from build123d import *

# Parameters (mm, degrees)
SKETCH1_R           = 1.5
SKETCH1_R_2         = 1
BOSS_EXTRUDE1_DEPTH = 4
FILLET1_R           = 10
FILLET2_R           = 10
FILLET3_R           = 10
FILLET4_R           = 10


with BuildPart() as part:
    # Sketch1 → Boss-Extrude1 (new body)
    with BuildSketch(Plane(origin=(0, 0, 0), x_dir=(1, 0, 0), z_dir=(0, 1, 0))):
        Polygon((-43.595803766, -205.807188304), (-22.135109681, -203.371959758), (-24.298008335, -184.311199966), (34.130185477, -177.681125241), (36.293084131, -196.741885032), (57.753778216, -194.306656487), (62.409879754, -235.339014996), (-38.939702228, -246.839546813), align=None)
        with Locations(Location((-29.093140713, -209.445179895, 0), (0, 0, 270))):
            Circle(SKETCH1_R, mode=Mode.SUBTRACT)
        with Locations(Location((44.434987391, -201.101656812, 0), (0, 0, 90))):
            Circle(SKETCH1_R, mode=Mode.SUBTRACT)
        with Locations(Location((11.278933321, -237.069365642, 0), (0, 0, 270))):
            Circle(SKETCH1_R, mode=Mode.SUBTRACT)
        with Locations(Location((-9.197768444, -205.174739373, 0), (0, 0, 270))):
            Circle(SKETCH1_R_2, mode=Mode.SUBTRACT)
        with Locations(Location((-11.22676603, -187.293996073, 0), (0, 0, 270))):
            Circle(SKETCH1_R_2, mode=Mode.SUBTRACT)
        with Locations(Location((22.059616288, -183.516860623, 0), (0, 0, 270))):
            Circle(SKETCH1_R_2, mode=Mode.SUBTRACT)
        with Locations(Location((24.088613874, -201.397603923, 0), (0, 0, 270))):
            Circle(SKETCH1_R_2, mode=Mode.SUBTRACT)
    extrude(amount=BOSS_EXTRUDE1_DEPTH)

    # Fillet1
    fillet1_edges = [part.edges().sort_by_distance(p)[0] for p in [
        (-38.939702228, 2, 246.839546813),
    ]]
    fillet(fillet1_edges, radius=FILLET1_R)

    # Fillet2
    fillet2_edges = [part.edges().sort_by_distance(p)[0] for p in [
        (62.409879754, 2, 235.339014996),
    ]]
    fillet(fillet2_edges, radius=FILLET2_R)

    # Fillet3
    fillet3_edges = [part.edges().sort_by_distance(p)[0] for p in [
        (57.753778216, 2, 194.306656487),
    ]]
    fillet(fillet3_edges, radius=FILLET3_R)

    # Fillet4
    fillet4_edges = [part.edges().sort_by_distance(p)[0] for p in [
        (-43.595803766, 2, 205.807188304),
    ]]
    fillet(fillet4_edges, radius=FILLET4_R)


solid = part.part
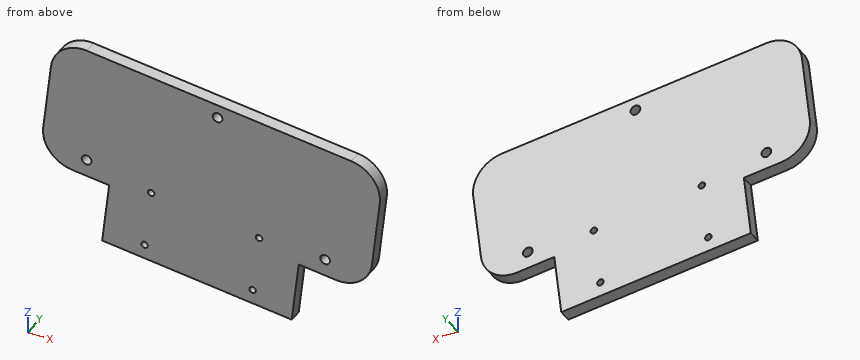
Part model, mm, in its own coordinate system. Coordinates: 2 decimals unless noted, no trailing zeros. Order: outer loops, then holes, each group sorted by start corner. A loop starts at its lowest first (then second) coordinate and runs counter-clockwise, first axis right, second up.
(1) Slice it at A-A, the plane y = 2.95. Write the cut outline in (x, z), and give its area (3 significant figures).
Check sheet entries:
outline: (-42.47, 215.74) arc R10 ccw to (-33.66, 204.68) - (-22.14, 203.37) - (-24.3, 184.31) - (34.13, 177.68) - (36.29, 196.74) - (47.82, 195.43) arc R10 ccw to (58.88, 204.24) - (61.28, 225.4) arc R10 ccw to (52.47, 236.47) - (-29, 245.71) arc R10 ccw to (-40.07, 236.9) - close; hole circle Ø3 at (-29.09, 209.45); hole circle Ø2 at (-11.23, 187.29); hole circle Ø2 at (-9.2, 205.17); hole circle Ø3 at (11.28, 237.07); hole circle Ø2 at (22.06, 183.52); hole circle Ø2 at (24.09, 201.4); hole circle Ø3 at (44.43, 201.1)
area: 5,220 mm2
(2) Pin check, flat tips, straight feed: pin 1 Ø1.5 at (y, z) = (2, 216) entering from -X; pin 2 Ø2 at (x, y) = (7, 1.5) entering from -Z; pin 3 Ø2 at (y, z) = (1, 221) entering from -X. Stop position of each tip, or through.
Check sheet entries:
pin 1: stops at x = -42.51
pin 2: stops at z = 180.65
pin 3: stops at x = -41.99
(3) Slice it at B-B, the plane z = 229. Write the cut outline in (x, y).
Check sheet entries:
outline: (-40.96, 0) - (61.04, 0) - (61.04, 4) - (-40.96, 4) - close
(4) Probe L1, parallel to Z at x = 22.5, y = 1.6; L2, parallel to Z at x = -10.5, y = 2.6; L3, parallel to X at y = 3.55, z = 200. List the from-to ranges inside material, lowest first.
Check sheet entries:
L1: z = 179 to 182.62, 184.41 to 239.87
L2: z = 182.75 to 186.61, 187.98 to 243.61
L3: x = -22.52 to 43.42, 45.45 to 57.38
(5) Slice it at C-C, the plane x = -35. Write the cut outline in (y, z), and give its area (3 significant figures).
Check sheet entries:
outline: (0, 204.93) - (4, 204.93) - (4, 244.51) - (0, 244.51) - close
area: 158 mm2
